```python
from build123d import *

# Parameters (mm, degrees)
F0_R     = 158
F1_DEPTH = 1400
F3_DEPTH = 158.001
F4_DEPTH = 158.001
F5_SIZE  = 137.99999
F6_SIZE  = 137.99999
F9_DEPTH = 80
F10_SIZE = 10
F11_SIZE = 10


# Not quite as in the source:
# - a fillet or chamfer is up to 0.001 mm smaller than in the source, because OpenCascade refuses the exact size


with BuildPart() as f1:
    # F0 (on Front) → F1 (new body)
    with BuildSketch(Plane.XZ):
        Circle(F0_R)
    extrude(amount=-F1_DEPTH)

    # F2 (on Right) → F3 (cut, through all)
    with BuildSketch(Plane.YZ):
        Polygon((167, 20), (390, 20), (455, 20), (455, 158), (167, 158), align=None)
        Polygon((945, 158), (945, 20), (1010, 20), (1233, 20), (1233, 158), align=None)
    extrude(amount=-F3_DEPTH, mode=Mode.SUBTRACT)

    # F4 (cut, through all): faces of the model
    f4_faces = [f1.faces().sort_by_distance(p)[0] for p in [
        (0, 1089, 89),
        (0, 311, 89),
    ]]
    extrude(f4_faces, amount=-F4_DEPTH, mode=Mode.SUBTRACT)

    # F5 (size 138 in the source; OpenCascade refuses exactly that, so slightly less here)
    f5_edges = [f1.edges().sort_by_distance(p)[0] for p in [
        (0, 1233, 20),
    ]]
    chamfer(f5_edges, length=F5_SIZE)

    # F6 (size 138 in the source; OpenCascade refuses exactly that, so slightly less here)
    f6_edges = [f1.edges().sort_by_distance(p)[0] for p in [
        (0, 167, 20),
    ]]
    chamfer(f6_edges, length=F6_SIZE)

    # F7 (on face) + F8 (on face) → F9 (cut)
    with BuildSketch(Plane.XY.offset(20)):
        Polygon((100, 1095), (0, 1095), (-100, 1095), (-100, 945), (100, 945), align=None)
    with BuildSketch(Plane.XY.offset(20)):
        Polygon((-100, 305), (0, 305), (100, 305), (100, 455), (-100, 455), align=None)
    extrude(amount=-F9_DEPTH, mode=Mode.SUBTRACT)

    # F10
    f10_edges = [f1.edges().sort_by_distance(p)[0] for p in [
        (-158, 0, 0),
        (-158, 1400, 0),
    ]]
    chamfer(f10_edges, length=F10_SIZE)

    # F11
    f11_edges = [f1.edges().sort_by_distance(p)[0] for p in [
        (0, 455, 158),
        (0, 945, 158),
    ]]
    chamfer(f11_edges, length=F11_SIZE)


solid = f1.part
```
Verification items for the finished model (mm, model axes). A direction names the side the tool comes from. Give positions to 0.01 mm unless a question says otherwise; leave off trailing zeros. Loops run counter-clockwise (first coordinate to the right, second up) from the corner with the lowest first, then second, coordinate; pieces in that order, holes last.
1. Mould release check, pull along Y, two halves, no side actions. Record for faces 4 (the flat face through (-2, 1400, 2)), 5 (the flat face through (-2, 0, 2)), 6 (the flat face through (-100, 381, -19)): released by +Y, released by -Y, zero draft, split by the parting line, or undercut.
2. Set-up check for faces 1 (the flat face through (-2, 1150, 75)), 2 (the flat face through (2, 945, 45)), 3 (the conical face through (-19.33, 0.486, 147.222)): record each of +Z, -Z, +X, -X, +Y, -Y from which the full face is reachable in a straight line by a thin tool's end or side.
3. Go/stop test with flat-tipped pins: pin 1 Ø12 at (x, y) = (10, 533.5) entering from -Z; pin 2 Ø1.5 at (y, z) = (783, -63.5) entering from -X; pin 3 Ø8 at (x, y) = (-117.5, 1073) entering from -Z. Record where each tip stops, or that it passes through.
4. Section check B-B, the plane y = 85. Enter the section's corners in (x, z).
5. Section check A-A, the plane z = 0. Enter the section's corners in (x, y).
6. Section check D-D, the plane y = 1050. Enter the section's corners in (x, z), then the cut area to 3 significant figures.
7. Section check C-C, the plane z = 82.5. Count the separate pieces of the cut face and the enclosed holes in it, then the cut area to 3 significant figures.
8. Thickness scan on line 1 (Y direction, x = -78, z = -53.5); line 2 (Y direction, x = -72.5, z = 39.5); line 3 (Z direction, x = -6.5, y = 1303.5). Record the ranges inside material, lowest first.
Geometry says:
1. face 4: released by +Y
1. face 5: released by -Y
1. face 6: undercut
2. face 1: +Z, +X, -X
2. face 2: +Z
2. face 3: -Y
3. pin 1: stops at z = -157.95
3. pin 2: stops at x = -145
3. pin 3: stops at z = -109.92
4. outline: circle Ø316 at (0, 0)
5. outline: (-158, 10) - (-148, 0) - (148, 0) - (158, 10) - (158, 1390) - (148, 1400) - (-148, 1400) - (-158, 1390) - close; hole (-100, 305) - (100, 305) - (100, 455) - (-100, 455) - close; hole (-100, 945) - (100, 945) - (100, 1095) - (-100, 1095) - close
6. outline: (-156.73, 20) arc R158 ccw (long way) to (156.73, 20) - (100, 20) - (100, -60) - (-100, -60) - (-100, 20) - close
6. area: 29,500 mm2
7. separate pieces: 3
7. enclosed holes: 0
7. area: 262,000 mm2
8. line 1: y = 0 to 305, 455 to 945, 1095 to 1400
8. line 2: y = 0 to 285.5, 455 to 945, 1114.5 to 1400
8. line 3: z = -157.87 to 157.87
